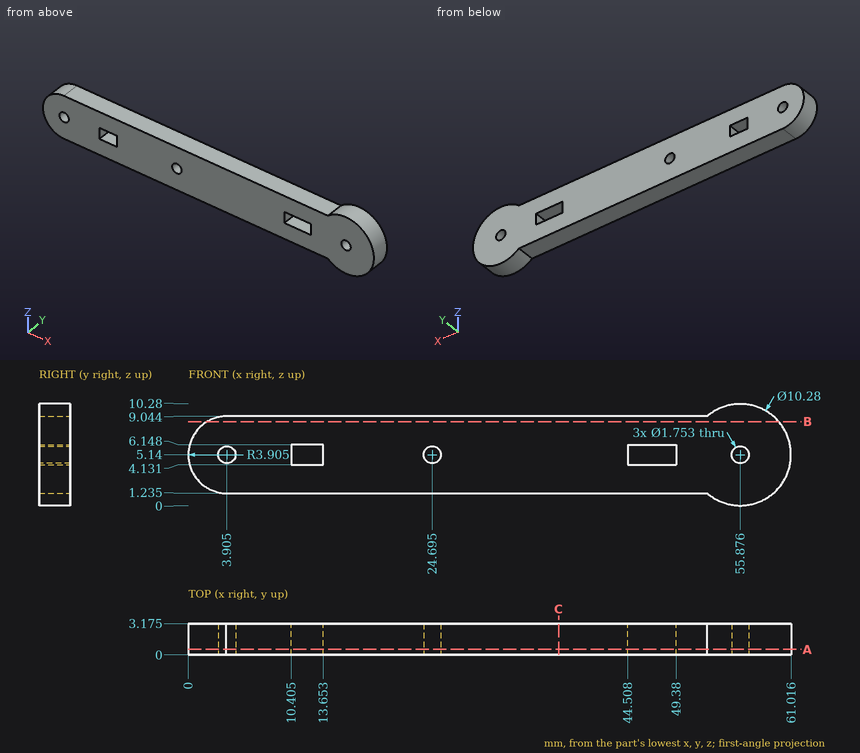
Geometry check sheet. Reference: drawing and pictorial views, mm from the part's lowest x, y, z. Coordinates: 2 decimals unless noted, no trailing zeros. Order: outer loops, then holes, each group sorted by start corner. A loop starts at its lowest first (then second) coordinate and runs counter-clockwise, first axis right, second up. Notation, with made-up numbers: (-5, 25.5) - (52, 25.5) arc R18 ccw to (52, 44.5) - close; hole circle Ø9 at (79, -23). An arc over 180 degrees is marked (long way). Answer in a Markdown table with one row per item. Add a question column.
1) Cross-section at B-B, the plane z = 8.5. Record the cut outline in (x, y) (1 decimal), then the cut area to 3 significant figures.
2) Cross-section at A-A, the plane y = 0.55. Record the cut outline in (x, z) (1 decimal), then the cut area to 3 significant figures.
3) Material ranges on line 1 along X through (y, z) = (3, 5.25) (1 decimal); line 2 along X through (y, z) = (0.8, 4.75) (1 decimal); line 3 along Z through (x, y) = (7.5, 2.1) (1 decimal), recorded low to high. Write a range as [from, to].
4) Cross-section at C-C, the plane x = 37.5. Record the cut outline in (y, z) (1 decimal).
5) Gauge pin test, flat ends, axial feed: P1, Ø1, axis at y = 1, z = 5, coming from the -X side; P2, Ø1.6, axis at x = 30.5, y = 2, coming from the +Z side; P3, Ø1, axis at x = 48, y = 1.5, coming from the -Z side (1 decimal). Record the tip position at first contact, or that the pin passes through.
Check result:
| question | item | result |
|---|---|---|
| 1 | outline | (1.9, 0) - (59.8, 0) - (59.8, 3.2) - (1.9, 3.2) - close |
| 1 | area | 184 mm² |
| 2 | outline | (3.9, 1.2) - (52.5, 1.2) arc R5.1 ccw (long way) to (52.5, 9) - (3.9, 9) arc R3.9 ccw to start; hole circle Ø1.8 at (3.9, 5.1); hole (10.4, 4.1) - (13.7, 4.1) - (13.7, 6.1) - (10.4, 6.1) - close; hole circle Ø1.8 at (24.7, 5.1); hole (44.5, 4.1) - (49.4, 4.1) - (49.4, 6.1) - (44.5, 6.1) - close; hole circle Ø1.8 at (55.9, 5.1) |
| 2 | area | 453 mm² |
| 3 | line 1 | x = [0, 3], [4.8, 10.4], [13.7, 23.8], [25.6, 44.5], [49.4, 55], [56.7, 61] |
| 3 | line 2 | x = [0, 3.1], [4.7, 10.4], [13.7, 23.9], [25.5, 44.5], [49.4, 55.1], [56.7, 61] |
| 3 | line 3 | z = [1.2, 9] |
| 4 | outline | (0, 1.2) - (3.2, 1.2) - (3.2, 9) - (0, 9) - close |
| 5 | P1 | stops at x = 0 |
| 5 | P2 | stops at z = 9.04 |
| 5 | P3 | stops at z = 1.2 |
